Geometry: final body of the model. Coordinates: model frame, mm. A direction names the side the tool comes from. Give positions to 0.01 mm unless a question says otherwise; leave off trailing zeros. Write each loop counter-clockwise with the first axis right and the second up, starting at its lowest first coordinate (ties: lowest second). Pieces come first, ordered by that corner, then holes.
from build123d import *

# Parameters (mm, degrees)
SKETCH1_R           = 45
SKETCH1_R_2         = 42.5
SKETCH1_R_3         = 3.5
BOSS_EXTRUDE1_DEPTH = 20
FILLET1_R           = 5
FILLET2_R           = 5
CUT_EXTRUDE2_DEPTH  = 6


with BuildPart() as part:
    # Sketch1 → Boss-Extrude1 (new body)
    # profile 1 of 2: a face of its own
    with BuildSketch(Plane.XY):
        Circle(SKETCH1_R)
        Circle(SKETCH1_R_2, mode=Mode.SUBTRACT)
    # profile 2 of 2: a face of its own
    with BuildSketch(Plane.XY):
        Circle(SKETCH1_R_2)
        Circle(SKETCH1_R_3, mode=Mode.SUBTRACT)
    extrude(amount=BOSS_EXTRUDE1_DEPTH)

    # Fillet1
    fillet1_edges = [part.edges().sort_by_distance(p)[0] for p in [
        (-45, 0, 0),
    ]]
    fillet(fillet1_edges, radius=FILLET1_R)

    # Fillet2
    fillet2_edges = [part.edges().sort_by_distance(p)[0] for p in [
        (-45, 0, 20),
    ]]
    fillet(fillet2_edges, radius=FILLET2_R)

    # Sketch2 → Cut-Extrude2 (cut)
    with BuildSketch(Plane(origin=(0, 0, 0), x_dir=(-1, 0, 0), z_dir=(0, 0, -1))):
        with BuildLine():
            Line((38.042260652, 12.360679775), (4.755282581, 1.545084972))
            ThreePointArc((4.755282581, 1.545084972), (4.938441703, 0.782172325), (5, 0))
            ThreePointArc((5, 0), (4.999202336, -0.08930847), (4.996809599, -0.178588445))
            Line((4.996809599, -0.178588445), (39.974476791, -1.42870756))
            Line((39.974476791, -1.42870756), (38.042260652, 12.360679775))
        make_face()
        with BuildLine():
            Line((38.042260652, -12.360679775), (4.755282581, -1.545084972))
            ThreePointArc((4.755282581, -1.545084972), (4.4137767, -2.349164796), (3.937532229, -3.081532078))
            Line((3.937532229, -3.081532078), (31.500257831, -24.652256622))
            Line((31.500257831, -24.652256622), (38.042260652, -12.360679775))
        make_face()
        with BuildLine():
            Line((23.511410092, -32.360679775), (2.938926261, -4.045084972))
            ThreePointArc((2.938926261, -4.045084972), (2.190015937, -4.494867094), (1.374251379, -4.807435194))
            Line((1.374251379, -4.807435194), (10.994011035, -38.459481554))
            Line((10.994011035, -38.459481554), (23.511410092, -32.360679775))
        make_face()
        with BuildLine():
            ThreePointArc((0, -5), (-0.870256478, -4.923682937), (-1.713946788, -4.697061465))
            Line((-1.713946788, -4.697061465), (-13.711574304, -37.576491721))
            Line((-13.711574304, -37.576491721), (0, -40))
            Line((0, -40), (0, -5))
        make_face()
        with BuildLine():
            ThreePointArc((-2.938926261, -4.045084972), (-3.598120497, -3.471819248), (-4.147475537, -2.792569904))
            Line((-4.147475537, -2.792569904), (-33.179804299, -22.34055923))
            Line((-33.179804299, -22.34055923), (-23.511410092, -32.360679775))
            Line((-23.511410092, -32.360679775), (-2.938926261, -4.045084972))
        make_face()
        with BuildLine():
            ThreePointArc((-4.755282581, -1.545084972), (-4.951624782, -0.693838608), (-4.996809599, 0.178588445))
            Line((-4.996809599, 0.178588445), (-39.974476791, 1.42870756))
            Line((-39.974476791, 1.42870756), (-38.042260652, -12.360679775))
            Line((-38.042260652, -12.360679775), (-4.755282581, -1.545084972))
        make_face()
        with BuildLine():
            ThreePointArc((-4.755282581, 1.545084972), (-4.4137767, 2.349164796), (-3.937532229, 3.081532078))
            Line((-3.937532229, 3.081532078), (-31.500257831, 24.652256622))
            Line((-31.500257831, 24.652256622), (-38.042260652, 12.360679775))
            Line((-38.042260652, 12.360679775), (-4.755282581, 1.545084972))
        make_face()
        with BuildLine():
            ThreePointArc((-2.938926261, 4.045084972), (-2.190015937, 4.494867094), (-1.374251379, 4.807435194))
            Line((-1.374251379, 4.807435194), (-10.994011035, 38.459481554))
            Line((-10.994011035, 38.459481554), (-23.511410092, 32.360679775))
            Line((-23.511410092, 32.360679775), (-2.938926261, 4.045084972))
        make_face()
        with BuildLine():
            Line((23.511410092, 32.360679775), (2.938926261, 4.045084972))
            ThreePointArc((2.938926261, 4.045084972), (3.598120497, 3.471819248), (4.147475537, 2.792569904))
            Line((4.147475537, 2.792569904), (33.179804299, 22.34055923))
            Line((33.179804299, 22.34055923), (23.511410092, 32.360679775))
        make_face()
        Polygon((13.711574304, 37.576491721), (1.713946788, 4.697061465), (0, 5), (0, 40), align=None)
    extrude(amount=-CUT_EXTRUDE2_DEPTH, mode=Mode.SUBTRACT)


solid = part.part
Q1. Pull-direction query (X, two-part tool) for faces 3 (the flat face through (13.37, -18.4, 2.96)), 4 (the flat face through (3, -3, 0)), 5 (the flat face through (24, 11, 6)); classes: released by +X, released by -X, zero draft, split by the parting line, or undercut.
Filled sheet:
face 3: undercut
face 4: zero draft
face 5: undercut
Q2. Access query for faces 1 (the flat face through (8, 1, 20)), 2 (the flat face through (-6.8, 38.8, 3)). Directions: +Z, -Z, +X, -X, +Y, -Y. A direction counts if a zero-diameter tool reaches every point of the face in a straight line with its end or side. Return the directions, or none.
Filled sheet:
face 1: +Z, +X, -X, +Y, -Y
face 2: -Z
Q3. Ray query, line 1 along Y through (x, z) = (-15, 1.5); line 2 along Y through (x, z) = (0, 12.25); line 3 along Y through (x, z) = (21.5, 4.25). Return the intervals inside material, ascending.
Filled sheet:
line 1: y = -40.91 to -36.51, -20.65 to -11.74, -4.87 to -0.54, 4.87 to 10.1, 20.65 to 40.91
line 2: y = -45 to -3.5, 3.5 to 45
line 3: y = -39.47 to -29.59, -14.48 to -6.99, 0.77 to 6.99, 16.83 to 29.59, 33.34 to 39.47
Q4. Section A-A on z = 18.5. Output: boundary loops of the cut face in (x, y).
Filled sheet:
outline: circle Ø87.14 at (0, 0); hole circle Ø7 at (0, 0)
Q5. Pin query (flat end, axial travel): P1, Ø11, axis at x = -9.5, y = -23, coming from the -Z side; P2, Ø3, axis at x = 27.5, z = 16.5, coming from the -Y side; P3, Ø5, axis at x = 13.5, z = 16, coming from the +Y side; P4, Ø6.5, axis at y = 17.5, z = 3, coming from the -X side. Return the tip coordinate at first contact, or that it passes through.
Filled sheet:
P1: stops at z = 0
P2: stops at y = -36.54
P3: stops at y = 43.6
P4: stops at x = -42.54
